Source: three-view drawing plus pictorial views. Frame: mm from the lowest corner of the part. A direction names the side the tool comes from. Coordinates: 2 decimals unless noted, no trailing zeros. Write each loop counter-clockwise with the first axis right and the second up, starting at its lowest first coordinate (ties: lowest second). Pieces come first, ordered by that corner, then holes. Notation, with made-up numbers: M 18,6.25 L 64,6.25 A24 ccw 64,29.25 Z; hole C -40,-8 d9. An arc over 180 degrees is marked long. Write item = value, one per line. Start each with the question number.
Item 1: Pull-direction query (Z, two-part tool) for the marked faces 3, 4 and 5; classes: +Z half, -Z half, draft (parallel to the pull), parting line (faces both ways), or undercut.
Item 2: First-contact query: pin 1 Ø6.5 at (x, z) = (18.7, 5.11) entering from +Y; pin 2 Ø5 at (x, z) = (6.7, 17.11) entering from +Y; pin 3 Ø3 at (x, z) = (18, 14) entering from +Y (1 decimal); pin 4 Ø12 at (x, z) = (21.5, 17) entering from +Y. Flat tips, straight axial feed; report the tip coordinate or a pass-through.
Item 3: Reachability of the marked faces 1 and 2 from +Z, -Z, +X, -X, +Y, -Y: full face, straight path, thin tool, end or side. Return the list, or none.
Item 4: Section D-D on z = 10. Output: boundary loops of the cut face in (x, y) (1 decimal).
Item 5: Ray query, L1, parallel to Z at x = 18.7, y = 0.4; L2, parallel to Y at x = 6.7, z = 24.75; L3, parallel to Y at x = 22.5, z = 8.5 (1 decimal). Return the intervals inside material, ascending. Write a range as [from, to].
Item 6: Section A-A on x = 6.7. Give the number of separate pieces and of enclosed holes in the cut face.
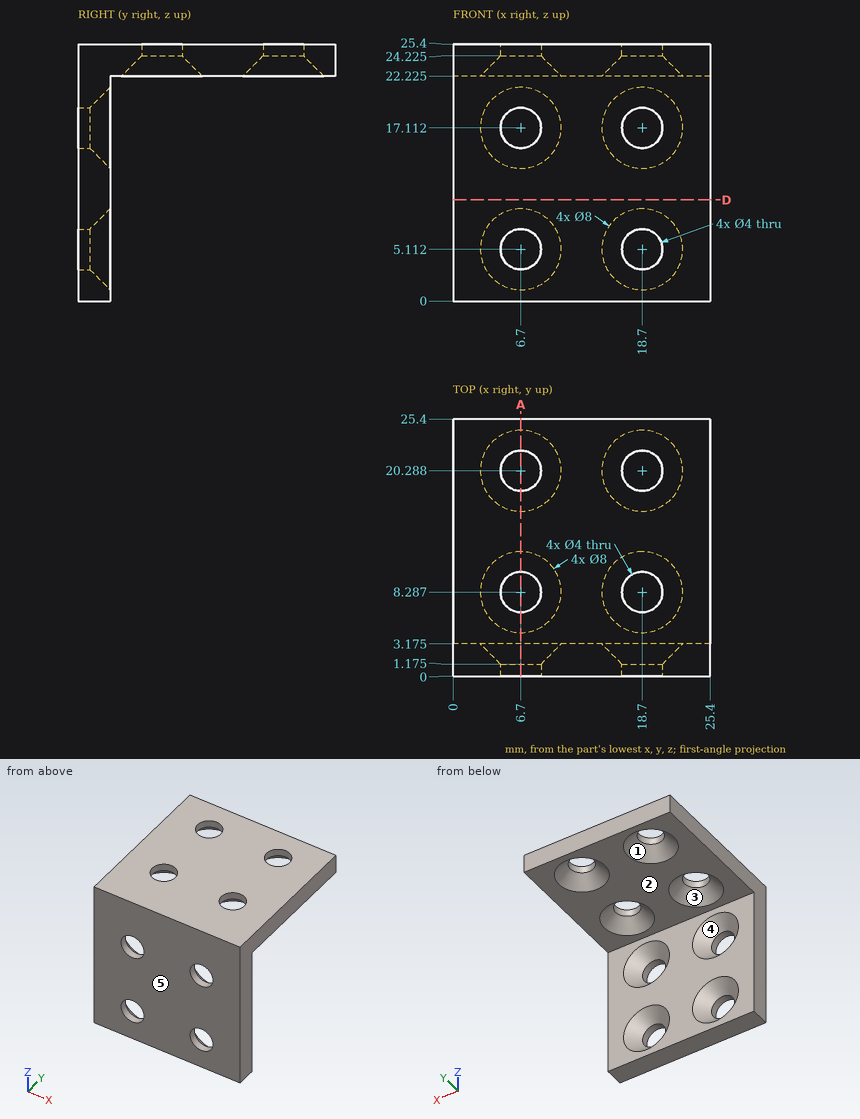
Responses:
q1.face_3 = -Z half
q1.face_4 = undercut
q1.face_5 = draft
q2.pin_1 = 2.43
q2.pin_2 = 1.68
q2.pin_3 = 3.2
q2.pin_4 = 25.4
q3.face_1 = -Z
q3.face_2 = -Z, +X, -X, +Y
q4.outline = M 0,0 L 25.4,0 L 25.4,3.2 L 0,3.2 Z
q5.L1 = [0, 3.11], [7.11, 15.11], [19.11, 25.4]
q5.L2 = [0, 6.29], [10.29, 18.29], [22.29, 25.4]
q5.L3 = [0, 3.2]
q6.separate_pieces = 5
q6.enclosed_holes = 0
